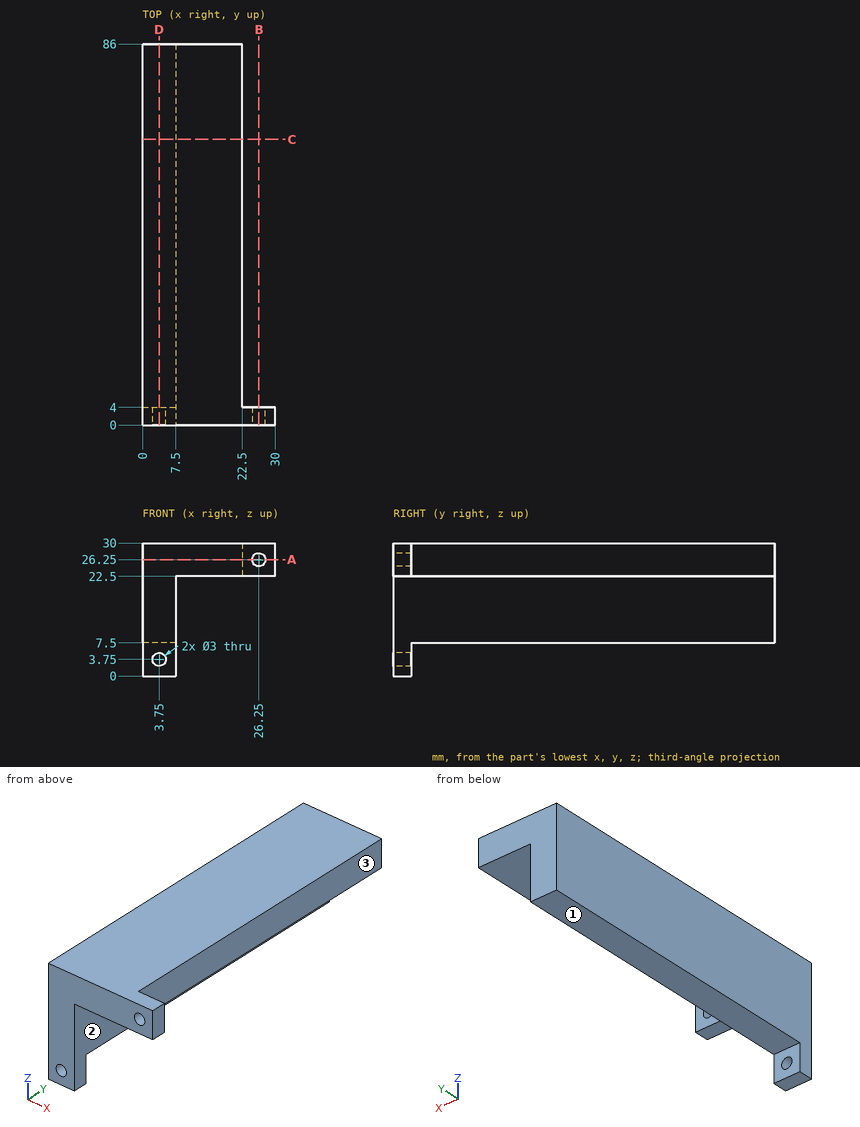
Study the drawing (mm; zero at the part's minimum x, y, z) and answer. A direction names the side the tool comes from. Give positions to 0.01 mm unless a question says otherwise; leave off trailing zeros. Order: outer loops, then holes, each group sorted by start corner. A loop starts at its lowest first (then second) coordinate and runs counter-clockwise, first axis right, second up.
1. Section B-B, the plane x = 26.25 is taken. Determine the outline of the cut face in (y, z), and give its area (3 significant figures).
Result sheet:
outline: (0, 22.5) - (4, 22.5) - (4, 24.75) - (0, 24.75) - close; (0, 27.75) - (4, 27.75) - (4, 30) - (0, 30) - close
area: 18.0 mm2
2. Each of these flat-tipped pins is pushed along its axis until it touches: P1, Ø18, axis at y = 51.5, z = 6.5, coming from the +X side; P2, Ø12, axis at y = 50, z = 17.5, coming from the -X side; P3, Ø4, axis at x = 25.5, z = 26, coming from the +Y side; P4, Ø8, axis at x = 4.5, y = 37, coming from the -Z side. Where does it stop, or does it pass through?
Result sheet:
P1: stops at x = 7.5
P2: stops at x = 0
P3: stops at y = 4
P4: stops at z = 7.5
3. Section C-C, the plane y = 64.5 is taken. Determine the outline of the cut face in (x, z).
Result sheet:
outline: (0, 7.5) - (7.5, 7.5) - (7.5, 22.5) - (22.5, 22.5) - (22.5, 30) - (0, 30) - close
4. Section A-A, the plane z = 26.25 is taken. Determine the outline of the cut face in (x, y).
Result sheet:
outline: (0, 0) - (24.75, 0) - (24.75, 4) - (22.5, 4) - (22.5, 86) - (0, 86) - close; (27.75, 0) - (30, 0) - (30, 4) - (27.75, 4) - close
5. For the marked faces 1, 2 and 3, determine the directions among +Z, -Z, +X, -X, +Y, -Y from which every point of the face is accessible in a straight line to the end or side of a thin tool.
Result sheet:
face 1: -Z, +X, -X, +Y
face 2: -Z, +X, +Y, -Y
face 3: +Z, -Z, +X, +Y
6. Straight lines are drawn through the part: L1, parallel to Z at x = 3.75, y = 3; L2, parallel to X at y = 2.8, z = 3.75; L3, parallel to Z at x = 26.25, y = 2.4. For each, find the intervals that lie inside material, in ascending order.
Result sheet:
L1: z = 0 to 2.25, 5.25 to 30
L2: x = 0 to 2.25, 5.25 to 7.5
L3: z = 22.5 to 24.75, 27.75 to 30
7. Section D-D, the plane x = 3.75 is taken. Determine the outline of the cut face in (y, z), and give its area (3 significant figures).
Result sheet:
outline: (0, 0) - (4, 0) - (4, 2.25) - (0, 2.25) - close; (0, 5.25) - (4, 5.25) - (4, 7.5) - (86, 7.5) - (86, 30) - (0, 30) - close
area: 1,950 mm2
